from build123d import *

# Parameters (mm, degrees)
F0_R           = 14.15
F0_R_2         = 1.5
F1_DEPTH       = 6
F2_R           = 20
F2_R_2         = 1.5
F3_DEPTH       = 3
F4_R           = 14
F4_R_2         = 1.5
F5_DEPTH       = 31
F6_R           = 4.5
F7_DEPTH       = 20.001
F7_DEPTH_BACK  = 20.001
F9_DEPTH       = 4.2
F11_DEPTH      = 20.001
F11_DEPTH_BACK = 20.001
F14_DEPTH      = 25
F17_DEPTH      = 25


with BuildPart() as f1:
    # F0 (on Top) → F1 (new body)
    with BuildSketch(Plane.XY):
        Circle(F0_R)
        Circle(F0_R_2, mode=Mode.SUBTRACT)
    extrude(amount=F1_DEPTH)

    # F2 (on face) → F3 (join)
    with BuildSketch(Plane.XY.offset(6)):
        Circle(F2_R)
        Circle(F2_R_2, mode=Mode.SUBTRACT)
    extrude(amount=F3_DEPTH)

    # F4 (on face) → F5 (join)
    with BuildSketch(Plane.XY.offset(9)):
        Circle(F4_R)
        Circle(F4_R_2, mode=Mode.SUBTRACT)
    extrude(amount=F5_DEPTH)

    # F6 (on Right) → F7 (cut, two sides)
    with BuildSketch(Plane.YZ) as f7_sk:
        with Locations((0, 26.5)):
            Circle(F6_R)
    extrude(amount=-F7_DEPTH, mode=Mode.SUBTRACT)
    extrude(f7_sk.sketch, amount=F7_DEPTH_BACK, mode=Mode.SUBTRACT)

    # F8 (on Right) → F9 (cut, symmetric)
    with BuildSketch(Plane.YZ):
        Polygon((-12.9903810568, 9.5), (12.9903810568, 9.5), (25.9807621135, 32), (25.9807621135, 52.7080496021), (-25.9807621135, 52.7080496021), (-25.9807621135, 32), align=None)
    extrude(amount=F9_DEPTH, both=True, mode=Mode.SUBTRACT)

    # F10 (on Right) → F11 (cut, two sides)
    with BuildSketch(Plane.YZ) as f11_sk:
        with BuildLine():
            Line((-3, 39.1491106407), (-3, 43.1880317001))
            Line((-3, 43.1880317001), (3, 43.1880317001))
            Line((3, 43.1880317001), (3, 39.1491106407))
            ThreePointArc((3, 39.1491106407), (10.1980390272, 34.5622577483), (13, 26.5))
            Line((13, 26.5), (13, 12.5))
            Line((13, 12.5), (19.3005313302, 12.5))
            Line((19.3005313302, 12.5), (19.3005313302, 47.1742767518))
            Line((19.3005313302, 47.1742767518), (-17.3973576033, 47.1742767518))
            Line((-17.3973576033, 47.1742767518), (-17.4070411782, 12.5))
            Line((-17.4070411782, 12.5), (-13, 12.5))
            Line((-13, 12.5), (-13, 26.5))
            ThreePointArc((-13, 26.5), (-10.1980390272, 34.5622577483), (-3, 39.1491106407))
        make_face()
    extrude(amount=-F11_DEPTH, mode=Mode.SUBTRACT)
    extrude(f11_sk.sketch, amount=F11_DEPTH_BACK, mode=Mode.SUBTRACT)

    # F13 (on offset) → F14 (cut)
    with BuildSketch(Plane.YZ.offset(11.5)):
        with BuildLine():
            Line((2.5, 32.5), (-2.5, 32.5))
            ThreePointArc((-2.5, 32.5), (-6.5, 26.5), (-2.5, 20.5))
            Line((-2.5, 20.5), (2.5, 20.5))
            ThreePointArc((2.5, 20.5), (6.5, 26.5), (2.5, 32.5))
        make_face()
    extrude(amount=F14_DEPTH, mode=Mode.SUBTRACT)

    # F16 (on offset) → F17 (cut)
    with BuildSketch(Plane.YZ.offset(-11.5)):
        with BuildLine():
            Line((2.5, 32.5), (-2.5, 32.5))
            ThreePointArc((-2.5, 32.5), (-6.5, 26.5), (-2.5, 20.5))
            Line((-2.5, 20.5), (2.5, 20.5))
            ThreePointArc((2.5, 20.5), (6.5, 26.5), (2.5, 32.5))
        make_face()
    extrude(amount=-F17_DEPTH, mode=Mode.SUBTRACT)


solid = f1.part
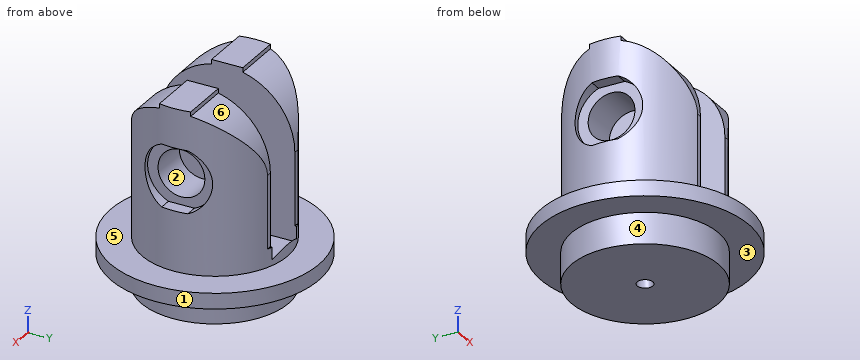
For this review, take the finished solid that the model builds, in its own axes (mm). Face numbers are marked on the shaded views. A direction names the side the tool comes from. Give positions to 0.01 mm unless a question says otherwise; leave off trailing zeros. Order: outer loops, then holes, each group sorted by start corner. A loop starts at its lowest first (then second) coordinate and runs counter-clockwise, first axis right, second up. Notation, with made-up numbers: M 18,-38.5 L 33,-38.5 A18 ccw 33,-5.5 Z; hole C -36,41.25 d7. An arc over 180 degrees is marked long. Answer in a Markdown table with one row per item. Add a question column.
(1) Consider section A-A on z = 18.5. State the section outline as (x, y) points.
(2) Mouldability with a two-part tool opening along Y and no side actions: class the marked faces 1, 2 and 3 as +Y half, -Y half, draft (parallel to the pull), parting line (faces both ways), or undercut.
(3) For pin 1 (6 mm diameter, centred on y = -5.5, z = 8.5, fed in from -X); pin 2 (6 mm diameter, centred on y = 5, z = 18, fed in from +X); pin 3 (10 mm diameter, centred on x = 9, z = 14.5, fed in from +Y), all flat-tipped, find the tip position at first contact; note any pin that passes through.
(4) Wall thickness on probe 1 along Z at (x, y) = (6.5, 0); probe 2 along Y at (x, z) = (0, 4); probe 3 along Z at (x, y) = (18.5, -2): over which ranges is each line inside the solid? List them lowest first. Write a range as [from, to].
(5) Consider section C-C on z = 29.5. State the section outline as (x, y) points.
(6) Consider section B-B on x = 0. State the section outline as (y, z) points, and give its area (3 significant figures).
(7) Consider section D-D on y = 0. Give the number of separate pieces and of enclosed holes in the cut face, and give its area (3 significant figures).
(8) For the marked faces 4, 5 and 6, list the 3-axis set-ups (+Z, -Z, +X, -X, +Y, -Y) from which the entire face can be reached by the end or side of a thin tool; tool diameter is ignored.
Evaluation:
| question | item | result |
|---|---|---|
| 1 | outline | M -5.2,-13 L -4.2,-13 L -4.2,13 L -5.2,13 A14 ccw Z; M 4.2,-13 L 5.2,-13 A14 ccw 5.2,13 L 4.2,13 Z |
| 2 | face 1 | parting line |
| 2 | face 2 | undercut |
| 2 | face 3 | draft |
| 3 | pin 1 | stops at x = -19.84 |
| 3 | pin 2 | stops at x = 13.86 |
| 3 | pin 3 | stops at y = 13.28 |
| 4 | probe 1 | z = [0, 22], [31, 40] |
| 4 | probe 2 | y = [-14.15, -1.5], [1.5, 14.15] |
| 4 | probe 3 | z = [6, 9] |
| 5 | outline | M -12.76,-5.77 A14 ccw -6,-12.65 L -4.2,-12.65 L -4.2,-3.35 L -11.5,-3.35 L -11.5,-5.77 Z; M -12.76,5.77 L -11.5,5.77 L -11.5,3.35 L -4.2,3.35 L -4.2,12.65 L -6,12.65 A14 ccw Z; M 4.2,-12.65 L 6,-12.65 A14 ccw 12.76,-5.77 L 11.5,-5.77 L 11.5,-3.35 L 4.2,-3.35 Z; M 4.2,3.35 L 11.5,3.35 L 11.5,5.77 L 12.76,5.77 A14 ccw 6,12.65 L 4.2,12.65 Z |
| 6 | outline | M -20,6 L -14.15,6 L -14.15,0 L -1.5,0 L -1.5,9.5 L -12.99,9.5 L -14,11.25 L -14,9 L -20,9 Z; M 1.5,0 L 14.15,0 L 14.15,6 L 20,6 L 20,9 L 14,9 L 14,11.25 L 12.99,9.5 L 1.5,9.5 Z |
| 6 | area | 277 mm^2 |
| 7 | separate pieces | 4 |
| 7 | enclosed holes | 0 |
| 7 | area | 682 mm^2 |
| 8 | face 4 | -Z |
| 8 | face 5 | +Z |
| 8 | face 6 | +Z, +X, -X, +Y |
